The model under review builds one solid part; all positions refer to its coordinate system, in mm. A direction names the side the tool comes from. Round coordinates to 2 decimals unless told otherwise and drop trailing zeros. Write each loop counter-clockwise with the first axis right and the second up, starting at its lowest first coordinate (ties: lowest second). Pieces come first, ordered by that corner, then holes. Notation, with made-up numbers: (27.5, 89) -> (52.5, 89) arc R15 cw to (52.5, 97) -> close; hole circle Ø4 at (-17.75, 44.5). An arc over 180 degrees is marked (long way). Use CSV: the item, a comma, the result in double quotes. Start each with the question number.
1) Take a section at A-A, the plane z = 0. Give the boundary of the cut face in (x, y).
2) For pin 1 Ø1.5 at (x, z) = (0, -1) entering from -Y; pin 2 Ø2 at (y, z) = (2, 0) entering from -X, all flat-tipped, find the tip position at first contact; note any pin that passes through.
3) Take a section at B-B, the plane x = 0.6. Give the boundary of the cut face in (y, z), then the cut area to 3 significant figures.
4) Mouldability with a two-part tool opening along Y and no side actions: class faces 1 (the face through (2.01, 2.23, -1.54)), 2 (the face through (0, 4.5, 0)), 3 (the face through (0, 0, 0)) as released by +Y, released by -Y, zero draft, split by the parting line, or undercut.
5) Machinability: for faces 4 (the face through (2.365, 4.254, 2.599)), 5 (the face through (-2, 0.5, 2)), which of the approach directions +Z, -Z, +X, -X, +Y, -Y give a long, thin tool a straight path to every point of the face, cutting with its end or side? Answer none if there is none.
6) Wall thickness on probe 1 along Y at (x, z) = (2.3, 2.4); probe 2 along X at (y, z) = (2.8, -0.4); probe 3 along X at (y, z) = (2.25, 0.85): over which ranges is each line inside the solid? List them lowest first. Write a range as [from, to].
7) Take a section at C-C, the plane y = 3.5. Give the boundary of the cut face in (x, z), then the cut area to 3 significant figures.
from build123d import *

# Parameters (mm, degrees)
SKETCH1_W           = 5.3
SKETCH1_H           = 5.8
BOSS_EXTRUDE1_DEPTH = 0.5
SKETCH2_R           = 2.533399168
BOSS_EXTRUDE2_DEPTH = 3.5
SKETCH3_W           = 5.3
SKETCH3_H           = 5.8
BOSS_EXTRUDE3_DEPTH = 0.5
FILLET1_R           = 1


with BuildPart() as part:
    # Sketch1 → Boss-Extrude1 (new body)
    with BuildSketch(Plane(origin=(0, 0, 0), x_dir=(1, 0, 0), z_dir=(0, 1, 0))):
        Rectangle(SKETCH1_W, SKETCH1_H)
    extrude(amount=BOSS_EXTRUDE1_DEPTH)

    # Sketch2 → Boss-Extrude2 (add)
    with BuildSketch(Plane(origin=(0, 0.5, 0), x_dir=(-1, 0, 0), z_dir=(0, 1, 0))):
        Circle(SKETCH2_R)
    extrude(amount=BOSS_EXTRUDE2_DEPTH)

    # Sketch3 → Boss-Extrude3 (add)
    with BuildSketch(Plane(origin=(0, 4, 0), x_dir=(-1, 0, 0), z_dir=(0, 1, 0))):
        Rectangle(SKETCH3_W, SKETCH3_H)
    extrude(amount=BOSS_EXTRUDE3_DEPTH)

    # Fillet1
    fillet1_edges = [part.edges().sort_by_distance(p)[0] for p in [
        (-2.65, 4.25, -2.9),
        (-2.65, 4.25, 2.9),
        (2.65, 4.25, 2.9),
        (2.65, 4.25, -2.9),
        (2.65, 0.25, 2.9),
        (-2.65, 0.25, 2.9),
        (-2.65, 0.25, -2.9),
        (2.65, 0.25, -2.9),
    ]]
    fillet(fillet1_edges, radius=FILLET1_R)


solid = part.part
Values found:
1,outline,"(-2.65, 0) -> (2.65, 0) -> (2.65, 0.5) -> (2.53, 0.5) -> (2.53, 4) -> (2.65, 4) -> (2.65, 4.5) -> (-2.65, 4.5) -> (-2.65, 4) -> (-2.53, 4) -> (-2.53, 0.5) -> (-2.65, 0.5) -> close"
2,pin 1,"y = 0"
2,pin 2,"x = -2.53"
3,outline,"(0, -2.9) -> (0.5, -2.9) -> (0.5, -2.46) -> (4, -2.46) -> (4, -2.9) -> (4.5, -2.9) -> (4.5, 2.9) -> (4, 2.9) -> (4, 2.46) -> (0.5, 2.46) -> (0.5, 2.9) -> (0, 2.9) -> close"
3,area,"23.0 mm²"
4,face 1,"undercut"
4,face 2,"released by +Y"
4,face 3,"released by -Y"
5,face 4,"+Z, +X, +Y, -Y"
5,face 5,"none"
6,probe 1,"[0, 0.5], [4, 4.5]"
6,probe 2,"[-2.5, 2.5]"
6,probe 3,"[-2.39, 2.39]"
7,outline,"circle Ø5.07 at (0, 0)"
7,area,"20.2 mm²"
